Read the model definition and answer for the solid it produces. Units are mm, in the model's axes. A direction names the side the tool comes from. Coordinates: 2 decimals unless noted, no trailing zeros. Write each loop counter-clockwise with the first axis right and the second up, starting at its lowest first coordinate (ties: lowest second). Pieces come first, ordered by that corner, then holes. Notation, with made-up numbers: (31.5, 54) -> (68.5, 54) arc R11 ccw to (68.5, 71) -> close; hole circle Ø8 at (37, -20). An arc over 180 degrees is marked (long way). Use CSV: the item, a comma, the result in double quotes.
from build123d import *

# Parameters (mm, degrees)
SKETCH1_W                       = 50.8
SKETCH1_H                       = 25.4
SKETCH1_W_2                     = 44.45
SKETCH1_H_2                     = 19.05
EXTRUDE_THIN1_DEPTH             = 228.6
F_1_8_0_13_DIAMETER_HOLE1_D     = 3.302
F_1_8_0_13_DIAMETER_HOLE1_DEPTH = 3.175
F_10_CLEARANCE_HOLE1_D          = 5.1054
F_10_0_2_DIAMETER_HOLE1_D       = 5.08
F_10_CLEARANCE_HOLE2_D          = 5.1054
F_10_CLEARANCE_HOLE2_DEPTH      = 3.175


with BuildPart() as part:
    # Sketch1 → Extrude-Thin1 (new body)
    with BuildSketch(Plane(origin=(0, 0, 0), x_dir=(0, 0, -1), z_dir=(1, 0, 0))):
        Rectangle(SKETCH1_W, SKETCH1_H)
        Rectangle(SKETCH1_W_2, SKETCH1_H_2, mode=Mode.SUBTRACT)
    extrude(amount=EXTRUDE_THIN1_DEPTH)

    # 1/8 (0.13) Diameter Hole1
    with Locations(Plane(origin=(0, -12.7, 0), x_dir=(-1, 0, 0), z_dir=(0, -1, 0))):
        with Locations((-190.5, -15.875), (-38.1, -15.875), (-63.5, 15.875), (-88.9, -15.875), (-114.3, 15.875), (-139.7, -15.875), (-165.1, 15.875)):
            Hole(F_1_8_0_13_DIAMETER_HOLE1_D / 2, depth=F_1_8_0_13_DIAMETER_HOLE1_DEPTH)

    # #10 Clearance Hole1 (through all)
    with Locations(Plane(origin=(0, 12.7, 0), x_dir=(1, 0, 0), z_dir=(0, 1, 0))):
        with Locations((82.55, 12.7), (82.55, 0), (82.55, -12.7), (146.05, -12.7), (146.05, 0), (146.05, 12.7)):
            Hole(F_10_CLEARANCE_HOLE1_D / 2)

    # #10 (0.2) Diameter Hole1 (through all)
    with Locations(Plane.XY.offset(25.4)):
        with Locations((12.7, 0), (215.9, 0)):
            Hole(F_10_0_2_DIAMETER_HOLE1_D / 2)

    # #10 Clearance Hole2
    with Locations(Plane(origin=(0, -12.7, 0), x_dir=(-1, 0, 0), z_dir=(0, -1, 0))):
        with Locations((-215.9, 12.7), (-215.9, 0), (-215.9, -12.7), (-12.7, -12.7), (-12.7, 0), (-12.7, 12.7)):
            Hole(F_10_CLEARANCE_HOLE2_D / 2, depth=F_10_CLEARANCE_HOLE2_DEPTH)


solid = part.part
1. A cutting plane is placed at A-A (x = 12.7). Give the vertices of the cut face in (y, z) (3 decimals), and give its area (3 significant figures).
Solutions:
outline,"(-12.7, -25.4) -> (-2.54, -25.4) -> (-2.54, -22.225) -> (-9.525, -22.225) -> (-9.525, -15.253) -> (-12.7, -15.253) -> close; (-12.7, -10.147) -> (-9.525, -10.147) -> (-9.525, -2.553) -> (-12.7, -2.553) -> close; (-12.7, 2.553) -> (-9.525, 2.553) -> (-9.525, 10.147) -> (-12.7, 10.147) -> close; (-12.7, 15.253) -> (-9.525, 15.253) -> (-9.525, 22.225) -> (-2.54, 22.225) -> (-2.54, 25.4) -> (-12.7, 25.4) -> close; (2.54, -25.4) -> (12.7, -25.4) -> (12.7, 25.4) -> (2.54, 25.4) -> (2.54, 22.225) -> (9.525, 22.225) -> (9.525, -22.225) -> (2.54, -22.225) -> close"
area,"363 mm^2"
2. Find the intervals of material crossed by line 1 along X through (y, z) = (11.9, 12.7); line 2 along X through (y, z) = (-11.5, 12.7); line 3 along Z through (x, y) = (146.05, -10.6), in increasing order.
Solutions:
line 1,"x = 0 to 80, 85.1 to 143.5, 148.6 to 228.6"
line 2,"x = 0 to 10.15, 15.25 to 80, 85.1 to 143.5, 148.6 to 213.35, 218.45 to 228.6"
line 3,"z = -25.4 to -15.25, -10.15 to -2.55, 2.55 to 10.15, 15.25 to 25.4"
3. A tool of negligible diameter and unlimited length cuts with its end or side. For faces 4 (the flat face through (113, 0, 22.225)), 5 (the cylindrical face through (85.1, 11.1, -12.8)), 6 (the cylindrical face through (15.058, -11.09, -11.722)), from which of +Z, -Z, +X, -X, +Y, -Y can it reach the whole face along a straight path? Write none if from no direction.
Solutions:
face 4,"+X, -X"
face 5,"+Y, -Y"
face 6,"-Y"
4. A cutting plane is placed at B-B (x = 82.55). Give the number of separate pieces and of enclosed holes in the cut face, and give its area (3 significant figures).
Solutions:
separate pieces,"6"
enclosed holes,"0"
area,"346 mm^2"
5. This flat-tipped pin is pushed along its axis until it touches: pin 1 Ø3 at (x, z) = (165.1, -15.875) entering from -Y (3 decimals). Where does it stop, or does it pass through?
Solutions:
pin 1,"stops at y = 9.525"
6. A cutting plane is placed at C-C (y = -6). Give the vertices of the cut face in (x, z) (3 decimals).
Solutions:
outline,"(0, -25.4) -> (228.6, -25.4) -> (228.6, -22.225) -> (0, -22.225) -> close; (0, 22.225) -> (228.6, 22.225) -> (228.6, 25.4) -> (0, 25.4) -> close"
7. For a pull along X with two mould halves and no side action, classify faces 1 (the flat face through (113, 9.525, 0)), 2 (the flat face through (228.6, 10, 0)), 3 (the cylindrical face through (218.438, 0.112, -23.835)) as pulls with the +X half, pulls with the -X half, needs draft (parallel to the pull), parting line crosses it, or undercut.
Solutions:
face 1,"needs draft"
face 2,"pulls with the +X half"
face 3,"undercut"
